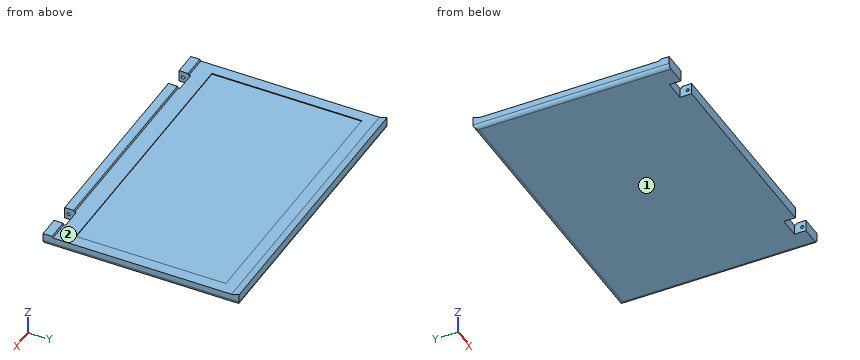
from build123d import *

# Parameters (mm, degrees)
BOSS_EXTRUDE1_DEPTH     = 375
SKETCH2_W               = 345
SKETCH2_H               = 195
CUT_EXTRUDE1_DEPTH      = 1
CHAMFER1_SIZE           = 5
CHAMFER1_SIZE_2         = 2.886751346
SKETCH3_W               = 27
SKETCH3_H               = 15
CUT_EXTRUDE2_DEPTH      = 30
CUT_EXTRUDE3_DEPTH      = 40
CUT_EXTRUDE3_DEPTH_BACK = 300
SKETCH4_R               = 2
BOSS_EXTRUDE2_DEPTH     = 375
FILLET1_R               = 5


with BuildPart() as part:
    # Sketch1 → Boss-Extrude1 (new body)
    with BuildSketch(Plane(origin=(0, 0, 0), x_dir=(0, 0, -1), z_dir=(1, 0, 0))):
        Polygon((0, 0), (-13, 0), (-15, 0), (-15, 10), (-13, 10), (-13, 255), (0, 255), align=None)
    extrude(amount=BOSS_EXTRUDE1_DEPTH)

    # Sketch2 → Cut-Extrude1 (cut)
    with BuildSketch(Plane.XY.offset(13)):
        with Locations((187.5, 132.5)):
            Rectangle(SKETCH2_W, SKETCH2_H)
    extrude(amount=-CUT_EXTRUDE1_DEPTH, mode=Mode.SUBTRACT)

    # Chamfer1
    # the kernel refuses this chamfer: 5, 2.886751346 mm, written as the material it adds along each edge
    with BuildSketch(Plane(origin=(0, 10, 13), x_dir=(0, -0.01932676561270064, 0.9998132206222079), z_dir=(1, 0, 0))) as chamfer1_piece_1_section:
        Polygon((CHAMFER1_SIZE * 0.999813220622, -CHAMFER1_SIZE * 0.0193267656127), (-CHAMFER1_SIZE_2 * 0.0193267656124, -CHAMFER1_SIZE_2 * 0.999813220604), (0, 0), align=None)
    chamfer1_piece_1 = extrude(amount=375, mode=Mode.PRIVATE)
    chamfer1_piece_1 = split(chamfer1_piece_1, bisect_by=Plane(origin=(187.5, 11.179939158, 15), z_dir=(0, 0, -1)), keep=Keep.TOP, mode=Mode.PRIVATE)
    add(chamfer1_piece_1)

    # Sketch3 → Cut-Extrude2 (cut)
    with BuildSketch(Plane.XY.offset(15)):
        with Locations((43.5, 7.5)):
            Rectangle(SKETCH3_W, SKETCH3_H)
        with Locations((333.5, 7.5)):
            Rectangle(SKETCH3_W, SKETCH3_H)
    extrude(amount=-CUT_EXTRUDE2_DEPTH, mode=Mode.SUBTRACT)

    # Sketch4 → Cut-Extrude3 (cut, two sides: drawn at the far end of the back side and taken through both)
    with BuildSketch(Plane.ZY.offset(-57).offset(-CUT_EXTRUDE3_DEPTH_BACK)):
        with Locations(Location((7, 5, 0), (0, 0, 180))):
            Circle(SKETCH4_R)
    extrude(amount=CUT_EXTRUDE3_DEPTH + CUT_EXTRUDE3_DEPTH_BACK, mode=Mode.SUBTRACT)

    # Sketch5 → Boss-Extrude2 (add)
    with BuildSketch(Plane(origin=(375, 0, 0), x_dir=(0, 0, -1), z_dir=(1, 0, 0))):
        Polygon((-13, 245), (-15.867453858, 255), (-13, 255), align=None)
    extrude(amount=-BOSS_EXTRUDE2_DEPTH)

    # Fillet1
    fillet1_edges = [part.edges().sort_by_distance(p)[0] for p in [
        (187.5, 255, 0),
        (375, 127.5, 0),
        (0, 127.5, 0),
    ]]
    fillet(fillet1_edges, radius=FILLET1_R)


solid = part.part
The model under review builds one solid part; all positions refer to its coordinate system, in mm. Face numbers are marked on the shaded views. Give positions to 0.01 mm unless a question says otherwise; leave off trailing zeros. Loops run counter-clockwise (first coordinate to the right, second up) from the corner with the lowest first, then second, coordinate; pieces in that order, holes last. Notation, with made-up numbers: (80.5, 26) -> (100.5, 26) arc R5 ccw to (100.5, 34) -> close; hole circle Ø8 at (37, 24.5). An arc over 180 degrees is marked (long way). Put each result on its own line as item: value. Start each with the question number.
1. Clearance check with flat-ended pins moving along their axes: P1, Ø8, axis at x = 44, y = 91, coming from the +Z side; P2, Ø3, axis at x = 252, z = 2.5, coming from the +Y side; P3, Ø4, axis at x = 336, z = 4, coming from the -Y side. State where each tip first meets the part, or that it passes through.
2. We need section A-A on x = 175. State the section outline as (y, z) points, then the cut area to 3 significant figures.
3. We need section B-B on y = 162.5. State the section outline as (x, z) points, then the cut area to 3 significant figures.
4. Wall thickness on probe 1 along Z at (x, y) = (25, 5); probe 2 along Y at (x, z) = (194.5, 7.5); probe 3 along Y at (x, z) = (354.75, 7): over which ranges is each line inside the solid? List them lowest first.
5. We need section C-C on y = 236.5. State the section outline as (x, z) points.
6. Mouldability with a two-part tool opening along Y and no side actions: class the marked faces 1 and 2 as released by +Y, released by -Y, zero draft, split by the parting line, or undercut.
Determined:
1. P1: z = 12
1. P2: y = 254.9
1. P3: y = 15
2. outline: (0, 0) -> (250, 0) arc R5 ccw to (255, 5) -> (255, 15.87) -> (245, 13) -> (230, 13) -> (230, 12) -> (35, 12) -> (35, 13) -> (12.89, 13) -> (11.73, 15) -> (0, 15) -> close; hole circle Ø4 at (5, 7)
2. area: 3,140 mm^2
3. outline: (0, 5) arc R5 ccw to (5, 0) -> (370, 0) arc R5 ccw to (375, 5) -> (375, 13) -> (360, 13) -> (360, 12) -> (15, 12) -> (15, 13) -> (0, 13) -> close
3. area: 4,520 mm^2
4. probe 1: 0 to 5, 9 to 15
4. probe 2: 0 to 3.06, 6.94 to 255
4. probe 3: 0 to 3, 7 to 255
5. outline: (0, 5) arc R5 ccw to (5, 0) -> (370, 0) arc R5 ccw to (375, 5) -> (375, 13) -> (0, 13) -> close
6. face 1: zero draft
6. face 2: undercut
